CAD build for the part. Positions are in the model's coordinates, mm. A direction names the side the tool comes from. Round coordinates to 2 decimals unless told otherwise and drop trailing zeros. Write each loop counter-clockwise with the first axis right and the second up, starting at its lowest first coordinate (ties: lowest second). Pieces come first, ordered by that corner, then holes. Notation, with made-up numbers: (29.5, 55.25) - (76.5, 55.25) arc R22 ccw to (76.5, 80.25) - close; hole circle Ø5 at (43, 88). An arc over 180 degrees is marked (long way). Answer in a Markdown table with one row per item.
Autodesk Inventor part; units mm, degrees
ref_plane "YZ Plane" through (0, 0, 0) normal (1, 0, 0) x (0, 1, 0)
ref_plane "XZ Plane" through (0, 0, 0) normal (0, 1, 0) x (-1, 0, 0)
ref_plane "XY Plane" through (0, 0, 0) normal (0, 0, 1) x (1, 0, 0)
sketch "Sketch1" plane through (0, 0, 0) normal (1, 0, 0) x (0, 1, 0)
  circle A0 centre (0, 0) radius 1.5
  circle A1 centre (0, 0) radius 3.5
  circle A2 centre (0, 0) radius 1.5
  line L0 (3.419, -0.7485) -> (3.9058, -0.7485)
  line L1 (3.9058, -0.7485) -> (3.9058, 0.7485)
  line L2 (3.9058, 0.7485) -> (3.419, 0.7485)
  line L3 (3.0942, -0.7485) -> (3.9058, 0.7485) construction
  line L4 (3.9058, -0.7485) -> (3.0942, 0.7485) construction
  point P0 (3.5, 0)
  dimension "d0" = 3
  dimension "d1" = 7
  dimension "d13" = 1.497
  dimension "d16" = 3
extrude "Extrusion1" add sketch "Sketch1" along normal blind 11 contours A0
extrude "Extrusion2" add sketch "Sketch1" against normal blind 1 contours A0 | A1
sketch "Sketch2" plane through (-1, 0, 0) normal (-1, 0, 0) x (0, 0, 1)
  point P0 (0, 0)
extrude "Extrusion3" add sketch "Sketch1" against normal blind 2 contours A0
sketch "Sketch3" plane through (-2, 0, 0) normal (-1, 0, 0) x (0, 0, 1)
  circle A0 centre (0, 0) radius 1
  dimension "d10" = 2
extrude "Extrusion4" cut sketch "Sketch3" against normal blind 1
extrude "Extrusion5" add sketch "Sketch1" against normal blind 1 contours A1 L2 L1 L0
properties material "Nickel-Copper Alloy 400"
Q1. Flat gauge pins, fed straight in: pin 1 (2 mm diameter, centred on x = 2, y = 3, fed in from -Z) (3 decimals); pin 2 (4 mm diameter, centred on x = 2.5, z = -3, fed in from -Y); pin 3 (0.5 mm diameter, centred on x = -0.5, y = 4, fed in from -Z). Where does each tip first touch, or does it go through?
Computed:
| item | result |
|---|---|
| pin 1 | passes through |
| pin 2 | stops at y = -1.12 |
| pin 3 | stops at z = -0.75 |
Q2. Saw through at A-A on y = 0. List the corners of the cut face in (x, z).
Computed:
| item | result |
|---|---|
| outline | (-2, -1.5) - (-1, -1.5) - (-1, -3.5) - (0, -3.5) - (0, -1.5) - (11, -1.5) - (11, 1.5) - (0, 1.5) - (0, 3.5) - (-1, 3.5) - (-1, 1.5) - (-2, 1.5) - (-2, 1) - (-1, 1) - (-1, -1) - (-2, -1) - close |
Q3. Drill centre lines: line 1 (X direction, y = -1, z = -3); line 2 (X direction, y = -0.75, z = 0.5); line 3 (Y direction, x = 4.25, z = -1.25). Where is each one in solid material? Low to high.
Computed:
| item | result |
|---|---|
| line 1 | x = -1 to 0 |
| line 2 | x = -1 to 11 |
| line 3 | y = -0.83 to 0.83 |
Q4. Saw through at B-B on z = 0. List the corners of the cut face in (x, y), then the cut area to 3 significant figures.
Computed:
| item | result |
|---|---|
| outline | (-2, -1.5) - (-1, -1.5) - (-1, -3.5) - (0, -3.5) - (0, -1.5) - (11, -1.5) - (11, 1.5) - (0, 1.5) - (0, 3.91) - (-1, 3.91) - (-1, 1.5) - (-2, 1.5) - (-2, 1) - (-1, 1) - (-1, -1) - (-2, -1) - close |
| area | 41.4 mm2 |
Q5. Saw through at C-C on x = -0.5. List the corners of the cut face in (y, z), then the cut area to 3 significant figures.
Computed:
| item | result |
|---|---|
| outline | (3.42, -0.75) - (3.91, -0.75) - (3.91, 0.75) - (3.42, 0.75) arc R3.5 ccw (long way) to start |
| area | 39.1 mm2 |
Q6. 3-axis set-ups, long thin cutter, end or side, ignore diameter. For faces 1 (the flat face through (-1, 0, -2)), 2 (the flat face through (11, 0, 0)), 3 (the cylindrical face through (5.42, -1.5, -0.07)): which of +Z, -Z, +X, -X, +Y, -Y reach the whole face in a straight line?
Computed:
| item | result |
|---|---|
| face 1 | -X |
| face 2 | +Z, -Z, +X, +Y, -Y |
| face 3 | +X |
Q7. Pull direction Z, two halves, no side cores. Call faces 4 (the cylindrical face through (-1.507, -0.976, -0.217)), 5 (the flat face through (0, 0, -2)), 6 (the flat face through (-1, 0, 0)), 7 (the cylindrical face through (-0.5, -3.5, 0.1)): released by +Z, released by -Z, zero draft, split by the parting line, or undercut.
Computed:
| item | result |
|---|---|
| face 4 | undercut |
| face 5 | zero draft |
| face 6 | undercut |
| face 7 | split by the parting line |
Q8. Saw through at D-D on y = 1.25. List the corners of the cut face in (x, z).
Computed:
| item | result |
|---|---|
| outline | (-2, -0.83) - (-1, -0.83) - (-1, -3.27) - (0, -3.27) - (0, -0.83) - (11, -0.83) - (11, 0.83) - (0, 0.83) - (0, 3.27) - (-1, 3.27) - (-1, 0.83) - (-2, 0.83) - close |
